Design review of the part shown in the three views and the two pictorial views. Dimensions are in mm from the part's minimum x, y and z. A direction names the side the tool comes from. Round coordinates to 2 decimals unless told otherwise and drop trailing zeros. Order: outer loops, then holes, each group sorted by start corner. A loop starts at its lowest first (then second) coordinate and runs counter-clockwise, first axis right, second up. Notation, with made-up numbers: (36, 12) -> (56, 12) arc R31 ccw to (56, 43) -> close; hole circle Ø10 at (3.25, 28.25). An arc over 180 degrees is marked (long way). Put each result on its own line as item: value. Start each with the question number.
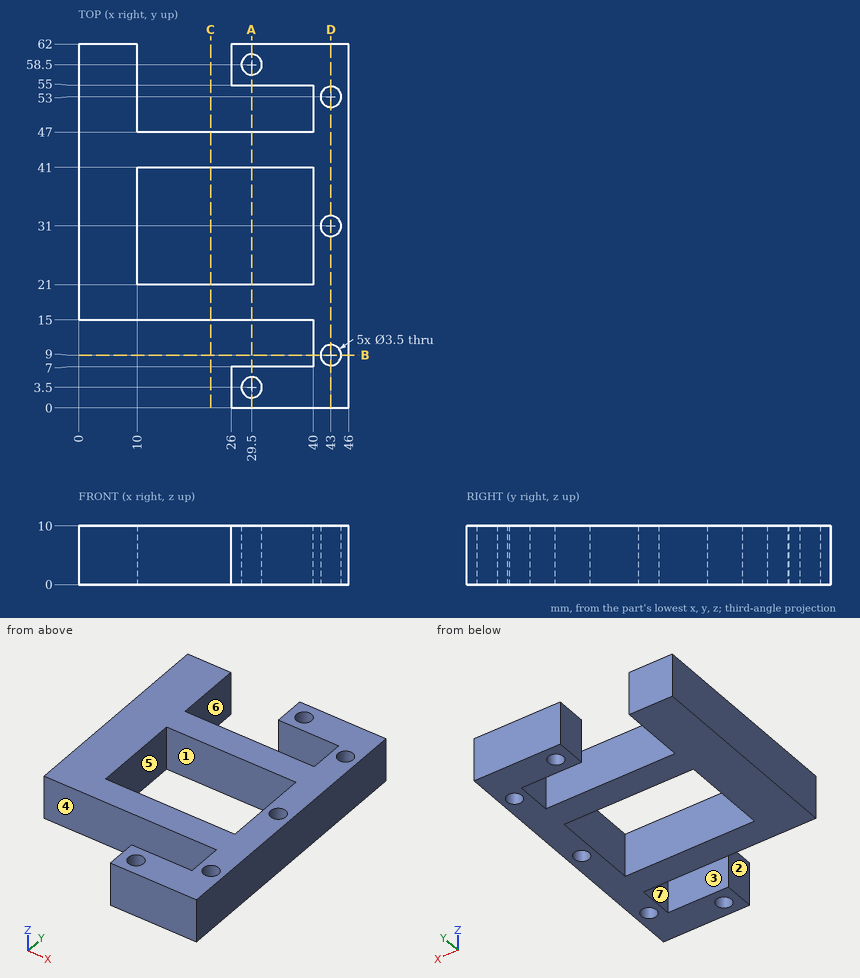
Q1. Take a section at A-A on x = 29.5. Give the boundary of the cut face in (y, z).
Q2. Draft analysis for pull direction X (two halves, no side actions). For the marked faces 4, 5, 6 and 7, state which applies: +X half, -X half, draft (parallel to the pull), parting line (faces both ways), or undercut.
Q3. For the marked faces 1, 2 and 3, list the 3-axis set-ups (+Z, -Z, +X, -X, +Y, -Y) from which the entire face can be reached by the end or side of a thin tool; tool diameter is ignored.
Q4. Take a section at D-D on x = 43. Give the boundary of the cut face in (y, z).
Q5. Take a section at B-B on y = 9. Give the boundary of the cut face in (x, z).
Q6. Take a section at C-C on x = 22.5. Give the boundary of the cut face in (y, z).
Q7. Clearance check with flat-ended pins moving along their axes: pin 1 Ø5 at (x, z) = (22.5, 7) entering from -Y; pin 2 Ø3.5 at (y, z) = (3, 7) entering from -X. State where each tip first meets the part, or that it passes through.
Q8. Wall thickness on probe 1 along Y at (x, z) = (27, 9.5); probe 2 along Y at (x, z) = (29.5, 3.25); probe 3 along Y at (x, z) = (43, 2.75): over which ranges is each line inside the solid? List them lowest first. Write a range as [from, to].
Calculated:
1. outline: (0, 0) -> (1.75, 0) -> (1.75, 10) -> (0, 10) -> close; (5.25, 0) -> (7, 0) -> (7, 10) -> (5.25, 10) -> close; (15, 0) -> (21, 0) -> (21, 10) -> (15, 10) -> close; (41, 0) -> (47, 0) -> (47, 10) -> (41, 10) -> close; (55, 0) -> (56.75, 0) -> (56.75, 10) -> (55, 10) -> close; (60.25, 0) -> (62, 0) -> (62, 10) -> (60.25, 10) -> close
2. face 4: draft
2. face 5: undercut
2. face 6: undercut
2. face 7: -X half
3. face 1: +Z, -Z
3. face 2: +Z, -Z, -X, -Y
3. face 3: +Z, -Z, -X
4. outline: (0, 0) -> (7.25, 0) -> (7.25, 10) -> (0, 10) -> close; (10.75, 0) -> (29.25, 0) -> (29.25, 10) -> (10.75, 10) -> close; (32.75, 0) -> (51.25, 0) -> (51.25, 10) -> (32.75, 10) -> close; (54.75, 0) -> (62, 0) -> (62, 10) -> (54.75, 10) -> close
5. outline: (40, 0) -> (41.25, 0) -> (41.25, 10) -> (40, 10) -> close; (44.75, 0) -> (46, 0) -> (46, 10) -> (44.75, 10) -> close
6. outline: (15, 0) -> (21, 0) -> (21, 10) -> (15, 10) -> close; (41, 0) -> (47, 0) -> (47, 10) -> (41, 10) -> close
7. pin 1: stops at y = 15
7. pin 2: stops at x = 26
8. probe 1: y = [0, 7], [15, 21], [41, 47], [55, 62]
8. probe 2: y = [0, 1.75], [5.25, 7], [15, 21], [41, 47], [55, 56.75], [60.25, 62]
8. probe 3: y = [0, 7.25], [10.75, 29.25], [32.75, 51.25], [54.75, 62]
